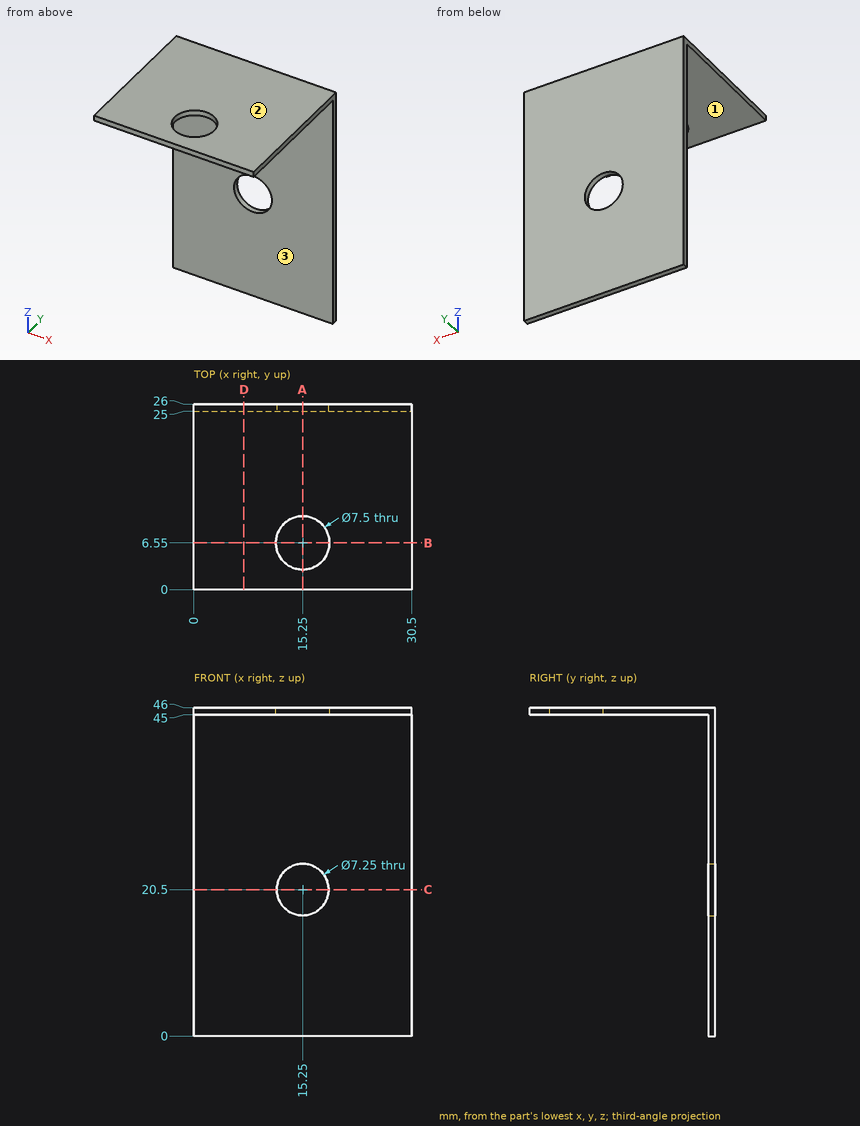
The figure shows three views and two pictorial views of one solid part (mm, origin at its lowest corner). Answer the questions. Give positions to 0.01 mm unless a question says otherwise; leave off trailing zeros. Order: outer loops, then holes, each group sorted by start corner. A loop starts at its lowest first (then second) coordinate and runs counter-clockwise, first axis right, second up. Notation, with made-up numbers: (43.25, 18) -> (55.25, 18) arc R6 cw to (55.25, 27) -> close; hole circle Ø8 at (64, 52.5). An arc over 180 degrees is marked (long way). Answer as a JSON object with one key per item and string values. Group by question number.
Item 1: The part is cut by section C-C on z = 20.5. Write down the section's boundary in (x, y) (3 decimals), and give its area (4 significant figures).
Item 2: Flat-ended cylindrical pins translate along their axes: pin 1 (5 mm diameter, centred on x = 19.5, z = 18, fed in from -Y); pin 2 (6.5 mm diameter, centred on x = 15.25, z = 20.5, fed in from +Y); pin 3 (1.5 mm diameter, centred on x = 5.5, y = 14, fed in from -Z). Find the tip coordinate at first contact, or state that the pin passes through.
Item 3: Determine the mould class of the marked faces 1, 2 and 3 for opening direction Z: pulls with the +Z half, pulls with the -Z half, needs draft (parallel to the pull), parting line crosses it, or undercut.
Item 4: Consider L1, parallel to Y at x = 15.25, z = 45.6; L2, parallel to Z at x = 15.25, y = 25.5 (3 decimals); L3, parallel to Y at x = 12.5, z = 7. Determine where each line is inside the solid, lowest interval first. Write a range as from..to.
Item 5: The part is cut by section A-A on x = 15.25. Write down the section's boundary in (y, z) (3 decimals).
Item 6: The part is cut by section D-D on x = 7. Write down the section's boundary in (y, z), and give its area (3 significant figures).
Item 7: The part is cut by section B-B on y = 6.55. Write down the section's boundary in (x, z), and give its area (3 significant figures).
Result set:
{
 "1": {"outline": "(0, 25) -> (11.625, 25) -> (11.625, 26) -> (0, 26) -> close; (18.875, 25) -> (30.5, 25) -> (30.5, 26) -> (18.875, 26) -> close", "area": "23.25 mm²"},
 "2": {"pin 1": "y = 25", "pin 2": "through", "pin 3": "z = 45"},
 "3": {"face 1": "pulls with the -Z half", "face 2": "pulls with the +Z half", "face 3": "needs draft"},
 "4": {"L1": "0..2.8, 10.3..26", "L2": "0..16.875, 24.125..46", "L3": "25..26"},
 "5": {"outline": "(0, 45) -> (2.8, 45) -> (2.8, 46) -> (0, 46) -> close; (10.3, 45) -> (25, 45) -> (25, 24.125) -> (26, 24.125) -> (26, 46) -> (10.3, 46) -> close; (25, 0) -> (26, 0) -> (26, 16.875) -> (25, 16.875) -> close"},
 "6": {"outline": "(0, 45) -> (25, 45) -> (25, 0) -> (26, 0) -> (26, 46) -> (0, 46) -> close", "area": "71.0 mm²"},
 "7": {"outline": "(0, 45) -> (11.5, 45) -> (11.5, 46) -> (0, 46) -> close; (19, 45) -> (30.5, 45) -> (30.5, 46) -> (19, 46) -> close", "area": "23.0 mm²"}
}
